The model under review builds one solid part; all positions refer to its coordinate system, in mm. Face numbers are marked on the shaded views. A direction names the side the tool comes from. Coordinates: 2 decimals unless noted, no trailing zeros. Loops run counter-clockwise (first coordinate to the right, second up) from the corner with the lowest first, then second, coordinate; pieces in that order, holes last. Notation, with made-up numbers: M -16,61 L -11,61 A17 cw -11,65 Z; hole C -26,79.5 d3. An arc over 180 degrees is marked long. One line per item, written item: value.
```python
from build123d import *

# Parameters (mm, degrees)
SKETCH2_R          = 2.25
SKETCH2_R_2        = 14.05
EXTRUDE6_DEPTH     = 30
SKETCH3_R          = 2.25
CUT_EXTRUDE1_DEPTH = 30
SKETCH4_W          = 30
SKETCH4_H          = 10
CUT_EXTRUDE2_DEPTH = 10


with BuildPart() as part:
    # Sketch2 → Extrude6 (new body)
    with BuildSketch(Plane.XY.offset(10)):
        Polygon((20, 0), (20, -36), (-20, -36), (-20, 36), (20, 36), align=None)
        with Locations((13.435028843, 13.435028843)):
            Circle(SKETCH2_R, mode=Mode.SUBTRACT)
        with Locations((0, 19)):
            Circle(SKETCH2_R, mode=Mode.SUBTRACT)
        with Locations((-13.435028843, 13.435028843)):
            Circle(SKETCH2_R, mode=Mode.SUBTRACT)
        with Locations((-13.435028843, -13.435028843)):
            Circle(SKETCH2_R, mode=Mode.SUBTRACT)
        with Locations((0, -19)):
            Circle(SKETCH2_R, mode=Mode.SUBTRACT)
        with Locations((13.435028843, -13.435028843)):
            Circle(SKETCH2_R, mode=Mode.SUBTRACT)
        Circle(SKETCH2_R_2, mode=Mode.SUBTRACT)
    extrude(amount=EXTRUDE6_DEPTH)

    # Sketch3 → Cut-Extrude1 (cut)
    with BuildSketch(Plane(origin=(20, 0, 0), x_dir=(0, 0, -1), z_dir=(1, 0, 0))):
        with Locations((-32.5, -31)):
            Circle(SKETCH3_R)
        with Locations((-17.5, -31)):
            Circle(SKETCH3_R)
        with Locations((-32.5, 31)):
            Circle(SKETCH3_R)
        with Locations((-17.5, 31)):
            Circle(SKETCH3_R)
    extrude(amount=-CUT_EXTRUDE1_DEPTH, mode=Mode.SUBTRACT)

    # Sketch4 → Cut-Extrude2 (cut)
    with BuildSketch(Plane.ZY.offset(20)):
        with Locations((25, 31)):
            Rectangle(SKETCH4_W, SKETCH4_H)
        with Locations((25, -31)):
            Rectangle(SKETCH4_W, SKETCH4_H)
    extrude(amount=-CUT_EXTRUDE2_DEPTH, mode=Mode.SUBTRACT)


solid = part.part
```
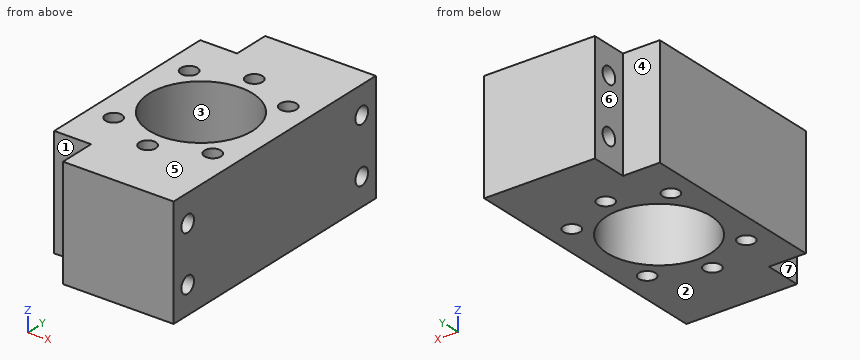
(1) Draft analysis for pull direction Y (two halves, no side actions). For the marked faces 1, 2, 3 and 4, state which applies: pulls with the +Y half, pulls with the -Y half, needs draft (parallel to the pull), parting line crosses it, or undercut.
Checks:
face 1: pulls with the -Y half
face 2: needs draft
face 3: undercut
face 4: pulls with the +Y half
(2) Add section C-C on x = 6. State the section outline as (y, z) points, then the cut area to 3 significant figures.
Checks:
outline: M -36,10 L -12.7,10 L -12.7,40 L -36,40 Z; M 12.7,10 L 36,10 L 36,40 L 12.7,40 Z; hole C -31,17.5 d4.5; hole C -31,32.5 d4.5; hole C 31,17.5 d4.5; hole C 31,32.5 d4.5
area: 1,330 mm^2
(3) Insertion check: pin 1 Ø5 at (x, y) = (-13.44, 13.44) entering from -Z; pin 2 Ø5 at (x, z) = (-16.5, 20) entering from +Y; pin 3 Ø8 at (x, z) = (-15.5, 24.5) entering from -Y; pin 4 Ø3.5 at (x, y) = (13.44, 13.44) entering from -Z. Each pin has a flat end and moves straight along its axis. Give the tip position at first contact, or say it passes through.
Checks:
pin 1: z = 10
pin 2: y = 26
pin 3: y = -26
pin 4: through
(4) Add section A-A on x = 0. State the section outline as (y, z) points.
Checks:
outline: M -36,10 L -21.25,10 L -21.25,40 L -36,40 Z; M -16.75,10 L -14.05,10 L -14.05,40 L -16.75,40 Z; M 14.05,10 L 16.75,10 L 16.75,40 L 14.05,40 Z; M 21.25,10 L 36,10 L 36,40 L 21.25,40 Z; hole C -31,17.5 d4.5; hole C -31,32.5 d4.5; hole C 31,17.5 d4.5; hole C 31,32.5 d4.5
(5) To check wall thickness, follow L1, parallel to Y at x = 0, z = 17.5; L2, parallel to Y at x = 6.5, z = 17.5; L3, parallel to X at y = -15.5, z = 23. State the ranges of each line that lie inside material, in increasing order. Write a range as [from, to].
Checks:
L1: [-36, -33.25], [-28.75, -21.25], [-16.75, -14.05], [14.05, 16.75], [21.25, 28.75], [33.25, 36]
L2: [-36, -33.25], [-28.75, -12.46], [12.46, 28.75], [33.25, 36]
L3: [-20, -14.33], [-12.54, 12.54], [14.33, 20]
(6) Add section D-D on y = 31. State the section outline as (x, z) points, then the cut area to 3 significant figures.
Checks:
outline: M -10,10 L 20,10 L 20,15.25 L -10,15.25 Z; M -10,19.75 L 20,19.75 L 20,30.25 L -10,30.25 Z; M -10,34.75 L 20,34.75 L 20,40 L -10,40 Z
area: 630 mm^2
(7) Add section B-B on y = 0. State the section outline as (x, z) points.
Checks:
outline: M -20,10 L -14.05,10 L -14.05,40 L -20,40 Z; M 14.05,10 L 20,10 L 20,40 L 14.05,40 Z
(8) Tool access review of the marked faces 5, 6 and 7: name each direction out of +Z, -Z, +X, -X, +Y, -Y from which nothing blocks a thin tool from reaching the whole face with its end or side.
Checks:
face 5: +Z, +X, -X, +Y, -Y
face 6: +Z, -Z, -X, +Y
face 7: +Z, -Z, -X, -Y
